The model under review builds one solid part; all positions refer to its coordinate system, in mm. Face numbers are marked on the shaded views. A direction names the side the tool comes from. Coordinates: 2 decimals unless noted, no trailing zeros. Write each loop counter-clockwise with the first axis right and the second up, starting at its lowest first coordinate (ties: lowest second). Pieces come first, ordered by that corner, then holes. Notation, with made-up numbers: (-0.75, 15.5) -> (39.25, 15.5) arc R5 ccw to (39.25, 19.5) -> close; hole circle Ø11 at (15.5, 0.25). An arc over 180 degrees is marked (long way). Write each question's results on one line, items separated by ' | '.
```python
from build123d import *

# Parameters (mm, degrees)
BOSS_EXTRUDE1_DEPTH        = 3
SKETCH2_W                  = 26
SKETCH2_H                  = 3
BOSS_EXTRUDE2_DEPTH        = 29.2
F_10_0_10_DIAMETER_HOLE1_D = 10
F_3_0_3_DIAMETER_HOLE1_D   = 3
F_10_0_10_DIAMETER_HOLE2_D = 10
F_3_0_3_DIAMETER_HOLE2_D   = 3
FILLET1_R                  = 2.5
FILLET3_R                  = 5


with BuildPart() as part:
    # Sketch1 → Boss-Extrude1 (new body)
    with BuildSketch(Plane(origin=(0, -13.75, 0), x_dir=(1, 0, 0), z_dir=(0, 1, 0))):
        with BuildLine():
            Line((13.000000223, -17.8), (13.000000223, 0))
            Line((13.000000223, 0), (-13, 0))
            Line((-13, 0), (-13, -17.8))
            ThreePointArc((-13, -17.8), (-9.198386918, -27.027675803), (1.11e-07, -30.899618316))
            ThreePointArc((1.11e-07, -30.899618316), (9.19838714, -27.027675803), (13.000000223, -17.8))
        make_face()
    extrude(amount=-BOSS_EXTRUDE1_DEPTH)

    # Sketch2 → Boss-Extrude2 (add)
    with BuildSketch(Plane(origin=(0, -13.75, 0), x_dir=(-1, 0, 0), z_dir=(0, 1, 0))):
        with Locations((0, 1.5)):
            Rectangle(SKETCH2_W, SKETCH2_H)
    extrude(amount=BOSS_EXTRUDE2_DEPTH)

    # Ø10.0 (10) Diameter Hole1 (through all)
    with Locations(Plane(origin=(0, -13.75, 0), x_dir=(1, 0, 0), z_dir=(0, 1, 0))):
        with Locations((-0.099999806, -19.5)):
            Hole(F_10_0_10_DIAMETER_HOLE1_D / 2)

    # Ø3.0 (3) Diameter Hole1 (through all)
    with Locations(Plane(origin=(0, -13.75, 0), x_dir=(1, 0, 0), z_dir=(0, 1, 0))):
        with Locations((8.5, -19.5), (-8.5, -19.5)):
            Hole(F_3_0_3_DIAMETER_HOLE1_D / 2)

    # Ø10.0 (10) Diameter Hole2 (through all)
    with Locations(Plane.XY.offset(3)):
        with Locations((0.1, 1.35)):
            Hole(F_10_0_10_DIAMETER_HOLE2_D / 2)

    # Ø3.0 (3) Diameter Hole2 (through all)
    with Locations(Plane.XY.offset(3)):
        with Locations((-7.8, 8.25), (8, -5.65), (-7.8, -5.65), (8, 8.25)):
            Hole(F_3_0_3_DIAMETER_HOLE2_D / 2)

    # Fillet1
    fillet1_edges = [part.edges().sort_by_distance(p)[0] for p in [
        (1.11e-07, -16.75, 0),
        (0, -13.75, 3),
    ]]
    fillet(fillet1_edges, radius=FILLET1_R)

    # Fillet3
    fillet3_edges = [part.edges().sort_by_distance(p)[0] for p in [
        (13, 15.45, 1.5),
        (-13, 15.45, 1.5),
    ]]
    fillet(fillet3_edges, radius=FILLET3_R)


solid = part.part
```
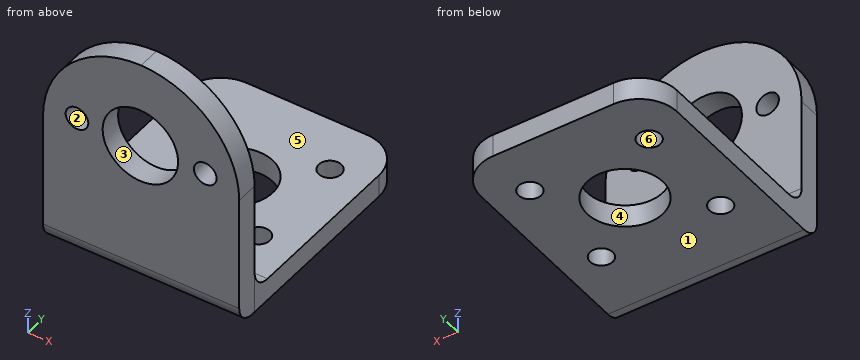
Q1. Add section C-C (z = 19.5). Write out the cut boundary in (x, y).
Solution:
outline: (-12.89, -16.75) -> (-10, -16.75) -> (-10, -13.75) -> (-12.89, -13.75) -> close; (-7, -16.75) -> (-5.1, -16.75) -> (-5.1, -13.75) -> (-7, -13.75) -> close; (4.9, -16.75) -> (7, -16.75) -> (7, -13.75) -> (4.9, -13.75) -> close; (10, -16.75) -> (12.89, -16.75) -> (12.89, -13.75) -> (10, -13.75) -> close
Q2. Clearance check with flat-ended pins moving along their axes: P1, Ø12, axis at x = -5.5, y = 9.5, coming from the +Z side; P2, Ø4, axis at x = 8.5, z = 19.5, coming from the +Y side. State where each tip first meets the part, or that it passes through.
Solution:
P1: z = 3 | P2: y = -13.75
Q3. Draft analysis for pull direction Z (two halves, no side actions). For the marked faces 1, 2, 3 and 4, state which applies: pulls with the +Z half, pulls with the -Z half, needs draft (parallel to the pull), parting line crosses it, or undercut.
Solution:
face 1: pulls with the -Z half | face 2: undercut | face 3: undercut | face 4: needs draft
Q4. Add section D-D (x = -3.75). Write out the cut boundary in (y, z).
Solution:
outline: (-16.75, 2.5) arc R2.5 ccw to (-14.25, 0) -> (-1.84, 0) -> (-1.84, 3) -> (-11.25, 3) arc R2.5 cw to (-13.75, 5.5) -> (-13.75, 16.08) -> (-16.75, 16.08) -> close; (-16.75, 22.92) -> (-13.75, 22.92) -> (-13.75, 30.32) -> (-16.75, 30.32) -> close; (4.54, 0) -> (15.45, 0) -> (15.45, 3) -> (4.54, 3) -> close
Q5. For line 1 (Y direction, x = -7.8, z = 0.7); line 2 (Y direction, x = 8, z = 0.85); line 3 (X direction, y = -15, z = 19.5), list the stretches that pass through material, from the lowest coordinate up. Write a range as from..to.
Solution:
line 1: -15.98..-7.15, -4.15..6.75, 9.75..15.45 | line 2: -16.13..-7.15, -4.15..6.75, 9.75..15.45 | line 3: -12.89..-10, -7..-5.1, 4.9..7, 10..12.89
Q6. Add section A-A (x = 8.5). Write out the cut boundary in (y, z).
Solution:
outline: (-16.75, 2.5) arc R2.5 ccw to (-14.25, 0) -> (-7.06, 0) -> (-7.06, 3) -> (-11.25, 3) arc R2.5 cw to (-13.75, 5.5) -> (-13.75, 18) -> (-16.75, 18) -> close; (-16.75, 21) -> (-13.75, 21) -> (-13.75, 27.68) -> (-16.75, 27.68) -> close; (-4.24, 0) -> (6.84, 0) -> (6.84, 3) -> (-4.24, 3) -> close; (9.66, 0) -> (15.42, 0) -> (15.42, 3) -> (9.66, 3) -> close
Q7. Machinability: for the marked faces 5 and 6, which of the approach directions +Z, -Z, +X, -X, +Y, -Y give a long, thin tool a straight path to every point of the face, cutting with its end or side? Answer none if there is none.
Solution:
face 5: +Z, +X, -X, +Y | face 6: +Z, -Z
Q8. Add section B-B (y = 5). Write out the cut boundary in (x, z), plus the area to 3 significant figures.
Solution:
outline: (-13, 0) -> (-3.32, 0) -> (-3.32, 3) -> (-13, 3) -> close; (3.52, 0) -> (13, 0) -> (13, 3) -> (3.52, 3) -> close | area: 57.5 mm²
